Work out the finished part from the listing and answer in its coordinate system (mm). A direction names the side the tool comes from. Coordinates: 2 decimals unless noted, no trailing zeros. Loops run counter-clockwise (first coordinate to the right, second up) from the corner with the lowest first, then second, coordinate; pieces in that order, holes last.
```python
from build123d import *

# Parameters (mm, degrees)
SKETCH_1_R          = 5
EXTRUDE_1_DEPTH     = 15
SKETCH_2_W          = 15
SKETCH_2_H          = 15
EXTRUDE_2_DEPTH     = 3
FILLET_1_R          = 2
SKETCH_3_W          = 15
SKETCH_3_H          = 15
SKETCH_3_W_2        = 10.2
SKETCH_3_H_2        = 10.2
EXTRUDE_3_DEPTH     = 32
CUT_EXTRUDE_1_DEPTH = 10
FILLET_2_R          = 1


with BuildPart() as part:
    # 草图1 → 凸台-拉伸1 (new body)
    with BuildSketch(Plane(origin=(0, 0, 0), x_dir=(1, 0, 0), z_dir=(0, 1, 0))):
        with Locations(Location((0, 0, 0), (0, 0, 270))):
            Circle(SKETCH_1_R)
    extrude(amount=EXTRUDE_1_DEPTH)

    # 草图2 → 凸台-拉伸2 (add)
    with BuildSketch(Plane(origin=(0, 15, 0), x_dir=(1, 0, 0), z_dir=(0, 1, 0))):
        Rectangle(SKETCH_2_W, SKETCH_2_H)
    extrude(amount=EXTRUDE_2_DEPTH)

    # 圆角1
    fillet_1_edges = [part.edges().sort_by_distance(p)[0] for p in [
        (0, 15, -5),
    ]]
    fillet(fillet_1_edges, radius=FILLET_1_R)

    # 草图3 → 凸台-拉伸3 (add)
    with BuildSketch(Plane(origin=(0, 18, 0), x_dir=(1, 0, 0), z_dir=(0, 1, 0))):
        Rectangle(SKETCH_3_W, SKETCH_3_H)
        Rectangle(SKETCH_3_W_2, SKETCH_3_H_2, mode=Mode.SUBTRACT)
    extrude(amount=EXTRUDE_3_DEPTH)

    # 草图4 → 切除-拉伸1 (cut)
    with BuildSketch(Plane.XZ):
        with BuildLine():
            Line((-1.85, 2.034698995), (-1.85, -2.034698995))
            ThreePointArc((-1.85, -2.034698995), (1.112429773, -2.514955268), (2.75, 0))
            ThreePointArc((2.75, 0), (1.112429773, 2.514955268), (-1.85, 2.034698995))
        make_face()
    extrude(amount=-CUT_EXTRUDE_1_DEPTH, mode=Mode.SUBTRACT)

    # 圆角2
    fillet_2_edges = [part.edges().sort_by_distance(p)[0] for p in [
        (-7.5, 15, 0),
        (-7.5, 32.5, -7.5),
        (0, 15, 7.5),
        (-7.5, 32.5, 7.5),
        (7.5, 15, 0),
        (7.5, 32.5, 7.5),
        (0, 15, -7.5),
        (7.5, 32.5, -7.5),
    ]]
    fillet(fillet_2_edges, radius=FILLET_2_R)


solid = part.part
```
1. For faces 4 (the cylindrical face through (-7.215, 15.301, -4.576)), 5 (the flat face through (-5.1, 34, 0)), 6 (the cylindrical face through (4.576, 15.301, -7.215)), 7 (the flat face through (-5.4, 15, 5.4)), determine the directions among +Z, -Z, +X, -X, +Y, -Y from which every point of the face is accessible in a straight line to the end or side of a thin tool.
2. A cutting plane is placed at B-B, the plane y = 4. Give the vertices of the cut face in (x, z).
3. Straight lines are drawn through the part: probe 1 along X at (y, z) = (22, -3.25); probe 2 along Y at (x, z) = (1, -1.25). For each, find the intervals that lie inside material, in ascending order.
4. A cutting plane is placed at A-A, the plane y = 29.5. Give the vertices of the cut face in (x, z).
5. Each of these flat-tipped pins is pushed along its axis until it touches: P1, Ø2, axis at x = 4.5, z = 5.5, coming from the -Y side; P2, Ø4, axis at y = 7.5, z = 0.5, coming from the +X side; P3, Ø3, axis at x = 2.5, y = 12.5, coming from the -Z side. Where does it stop, or does it pass through?
6. Determine the mould class of faces 1 (the flat face through (-1.85, 5, 0)), 2 (the cylindrical face through (-4.522, 15.301, -7.215)), 3 (the flat face through (-2.2, 0, -0.1)) for opening direction Z: released by +Z, released by -Z, zero draft, split by the parting line, or undercut.
Answers below:
1. face 4: -Z, -X, -Y
1. face 5: +Y
1. face 6: -Z, +X, -Y
1. face 7: +Z, -X, -Y
2. outline: circle Ø10 at (0, 0); hole (-1.85, -2.03) arc R2.75 ccw (long way) to (-1.85, 2.03) - close
3. probe 1: x = -7.5 to -5.1, 5.1 to 7.5
3. probe 2: y = 10 to 18
4. outline: (-7.5, -6.5) arc R1 ccw to (-6.5, -7.5) - (6.5, -7.5) arc R1 ccw to (7.5, -6.5) - (7.5, 6.5) arc R1 ccw to (6.5, 7.5) - (-6.5, 7.5) arc R1 ccw to (-7.5, 6.5) - close; hole (-5.1, -5.1) - (5.1, -5.1) - (5.1, 5.1) - (-5.1, 5.1) - close
5. P1: stops at y = 14.79
5. P2: stops at x = 5
5. P3: stops at z = -4.9
6. face 1: undercut
6. face 2: released by -Z
6. face 3: zero draft
